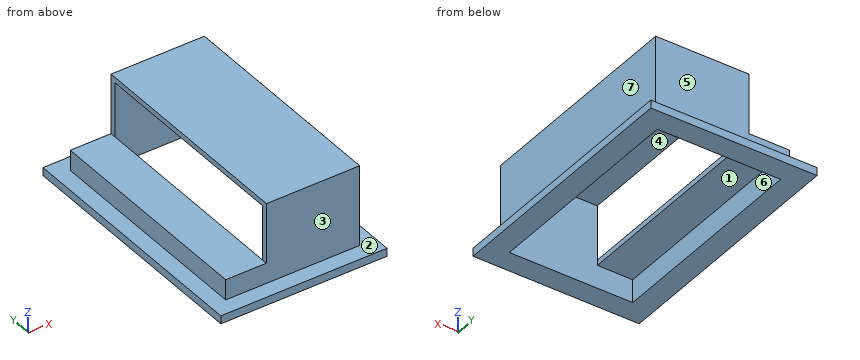
```python
from build123d import *

# Parameters (mm, degrees)
ESBO_O1_W                = 31
ESBO_O1_H                = 47.5
ESBO_O1_W_2              = 24
ESBO_O1_H_2              = 41.5
RESSALTO_EXTRUS_O1_DEPTH = 1.5
RESSALTO_EXTRUS_O2_DEPTH = 16.5
RESSALTO_EXTRUS_O3_START = 16.5
ESBO_O1_5_W              = 23
ESBO_O1_5_H              = 39.5
RESSALTO_EXTRUS_O3_DEPTH = 1
ESBO_O2_W                = 6.6
ESBO_O2_H                = 41.5
CORTE_EXTRUS_O1_DEPTH    = 15
RESSALTO_EXTRUS_O6_START = -1
RESSALTO_EXTRUS_O6_DEPTH = 39.5
ESBO_O4_W                = 3.8
ESBO_O4_H                = 1
RESSALTO_EXTRUS_O9_DEPTH = 7.6


with BuildPart() as part:
    # Esbo_o1 → Ressalto-extrus_o1 (new body)
    with BuildSketch(Plane.XY):
        with Locations((11.5, 20.75)):
            Rectangle(ESBO_O1_W, ESBO_O1_H)
        with Locations((12, 20.75)):
            Rectangle(ESBO_O1_W_2, ESBO_O1_H_2, mode=Mode.SUBTRACT)
    extrude(amount=RESSALTO_EXTRUS_O1_DEPTH)

    # Esbo_o1_4 → Ressalto-extrus_o2 (add)
    with BuildSketch(Plane.XY):
        Polygon((0, 41.5), (0, 40.5), (23, 40.5), (23, 1), (0, 1), (0, 0), (24, 0), (24, 41.5), align=None)
    extrude(amount=RESSALTO_EXTRUS_O2_DEPTH)

    # Esbo_o1_5 → Ressalto-extrus_o3 (add)
    with BuildSketch(Plane.XY.offset(RESSALTO_EXTRUS_O3_START)):
        with Locations((11.5, 20.75)):
            Rectangle(ESBO_O1_5_W, ESBO_O1_5_H)
    extrude(amount=-RESSALTO_EXTRUS_O3_DEPTH)

    # Esbo_o2 → Corte-extrus_o1 (cut)
    with BuildSketch(Plane.XY.offset(16.5)):
        with Locations((3.3, 20.75)):
            Rectangle(ESBO_O2_W, ESBO_O2_H)
    extrude(amount=-CORTE_EXTRUS_O1_DEPTH, mode=Mode.SUBTRACT)



with BuildPart() as body_2:
    # Esbo_o3 → Ressalto-extrus_o6 (new body)
    with BuildSketch(Plane(origin=(0, 41.5, 0), x_dir=(1, 0, 0), z_dir=(0, 1, 0)).offset(RESSALTO_EXTRUS_O6_START)):
        Polygon((-1, -1.5), (-1, -5.3), (6.6, -5.3), (6.6, -4.3), (0, -4.3), (0, -1.5), align=None)
    extrude(amount=-RESSALTO_EXTRUS_O6_DEPTH)


with BuildPart() as part_1:
    add(part.part)

    add(body_2.part)  # Ressalto-extrus_o9 merges body 2
    # Esbo_o4 → Ressalto-extrus_o9 (add)
    with BuildSketch(Plane.ZY.offset(-6.6)):
        with Locations((3.4, 41)):
            Rectangle(ESBO_O4_W, ESBO_O4_H)
        with Locations((3.4, 0.5)):
            Rectangle(ESBO_O4_W, ESBO_O4_H)
    extrude(amount=RESSALTO_EXTRUS_O9_DEPTH)


solid = part_1.part
```
CAD build for the part. Positions are in the model's coordinates, mm. Face numbers are marked on the shaded views. A direction names the side the tool comes from. Coordinates: 2 decimals unless noted, no trailing zeros. Order: outer loops, then holes, each group sorted by start corner. A loop starts at its lowest first (then second) coordinate and runs counter-clockwise, first axis right, second up. Notation, with made-up numbers: M 61,83 L 118,83 A24 ccw 118,101 Z; hole C 86.25,12.5 d3. An arc over 180 degrees is marked long. Write each question's results on one line, items separated by ' | '. Start each with the question number.
Q1. Cut at B-B (y = 15). List the corners of the cut face in (x, z).
Q2. Cut at D-D (z = 14.25). List the corners of the cut face in (x, y), then the cut area to 3 significant figures.
Q3. Cut at A-A (z = 3.25). List the corners of the cut face in (x, y), then the cut area to 3 significant figures.
Q4. Flat gauge pins, fed straight in: P1, Ø8, axis at y = 7.5, z = 7, coming from the +X side; P2, Ø1.5, axis at x = 15, z = 13, coming from the -Y side; P3, Ø1.1, axis at y = 30.5, z = 3, coming from the -X side. Where does each tip first touch, or does it go through?
Q5. Cut at C-C (x = 2.5). List the corners of the cut face in (y, z), then the cut area to 3 significant figures.
Q6. Which spindle directions (+Z, -Z, +X, -X, +Y, -Y) get a long thin tool onto all of the face, cutting with end or side? Do the marked faces 4, 5, 6 and 7. Say none if no direction does.
Q7. Drill centre lines: probe 1 along Y at (x, z) = (14.5, 3); probe 2 along X at (y, z) = (22, 1.25); probe 3 along Z at (x, y) = (1.5, 25.5). Where is each one in solid material? Low to high. Write a range as from..to.
Q8. Pull direction Y, two halves, no side cores. Call the marked faces 1, 2 and 3: +Y half, -Y half, draft (parallel to the pull), parting line (faces both ways), or undercut.
Found:
1) outline: M -4,0 L 0,0 L 0,4.3 L 6.6,4.3 L 6.6,5.3 L -1,5.3 L -1,1.5 L -4,1.5 Z; M 6.6,15.5 L 23,15.5 L 23,0 L 27,0 L 27,1.5 L 24,1.5 L 24,16.5 L 6.6,16.5 Z
2) outline: M 6.6,0 L 24,0 L 24,41.5 L 6.6,41.5 L 6.6,40.5 L 23,40.5 L 23,1 L 6.6,1 Z | area: 74.3 mm²
3) outline: M -1,0 L 24,0 L 24,41.5 L -1,41.5 Z; hole M 0,1 L 23,1 L 23,40.5 L 0,40.5 Z | area: 129 mm²
4) P1: x = 24 | P2: y = 0 | P3: x = -1
5) outline: M -3,0 L 1,0 L 1,4.3 L 40.5,4.3 L 40.5,0 L 44.5,0 L 44.5,1.5 L 41.5,1.5 L 41.5,5.3 L 0,5.3 L 0,1.5 L -3,1.5 Z | area: 59.1 mm²
6) face 4: -Z, -X | face 5: +Z, +X, -X, +Y | face 6: -Z | face 7: +Z, +X, +Y, -Y
7) probe 1: 0..1, 40.5..41.5 | probe 2: -4..0, 23..27 | probe 3: 4.3..5.3
8) face 1: undercut | face 2: draft | face 3: -Y half
